Model file for the job. Use its own axes, mm. Coordinates: 2 decimals unless noted, no trailing zeros. Write each loop counter-clockwise with the first axis right and the second up, starting at its lowest first coordinate (ties: lowest second). Pieces come first, ordered by that corner, then holes.
Q1. Pin check, flat tip, straight feed: P1, Ø1, axis at x = 8, z = -2, coming from the +Y side. Stop position of the tip, or through.
Q2. Drill centre lines: probe 1 along X at (y, z) = (-1.3, 0); probe 2 along Z at (x, y) = (40, -1.3); probe 3 along X at (y, z) = (-1.5, -2). Where is each one in solid material? Low to high.
Q3. Band-saw the part on A-A, the plane x = -40. Write the cut outline in (y, z), plus the area to 3 significant figures.
Q4. Band-saw the part on B-B, the plane z = 0. Write the cut outline in (x, y).
Q5. Band-saw the part on C-C, the plane y = -1.1. Write the cut outline in (x, z), plus the area to 3 significant figures.
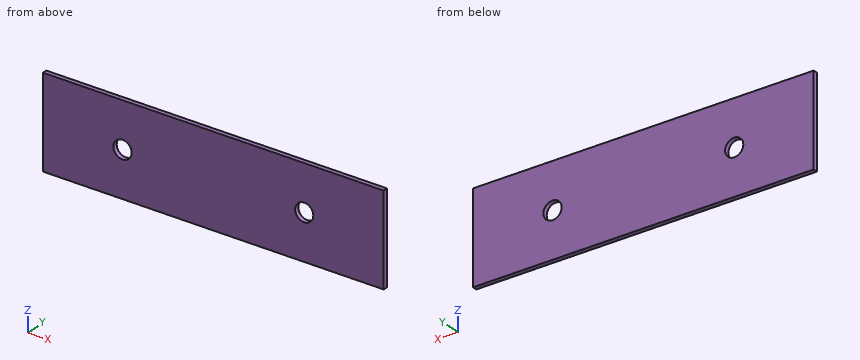
from build123d import *

# Parameters (mm, degrees)
SKETCH1_W          = 150
SKETCH1_H          = 40
BASE_FLANGE1_DEPTH = 2
SKETCH4_R          = 4
CUT_EXTRUDE1_DEPTH = 2


# Sheet-metal steps are written as plain solids
with BuildPart() as part:
    # Sketch1 → Base-Flange1 (new body)
    with BuildSketch(Plane(origin=(0, 0, 0), x_dir=(1, 0, 0), z_dir=(0, 1, 0))):
        Rectangle(SKETCH1_W, SKETCH1_H)
    extrude(amount=-BASE_FLANGE1_DEPTH)

    # Sketch4 → Cut-Extrude1 (cut)
    with BuildSketch(Plane(origin=(0, 0, 0), x_dir=(1, 0, 0), z_dir=(0, 1, 0))):
        with Locations(Location((-40, 0, 0), (0, 0, 270))):
            Circle(SKETCH4_R)
        with Locations(Location((40, 0, 0), (0, 0, 90))):
            Circle(SKETCH4_R)
    extrude(amount=-CUT_EXTRUDE1_DEPTH, mode=Mode.SUBTRACT)


solid = part.part
Answer sheet:
1. P1: stops at y = 0
2. probe 1: x = -75 to -44, -36 to 36, 44 to 75
2. probe 2: z = -20 to -4, 4 to 20
2. probe 3: x = -75 to -43.46, -36.54 to 36.54, 43.46 to 75
3. outline: (-2, -20) - (0, -20) - (0, -4) - (-2, -4) - close; (-2, 4) - (0, 4) - (0, 20) - (-2, 20) - close
3. area: 64.0 mm2
4. outline: (-75, -2) - (-44, -2) - (-44, 0) - (-75, 0) - close; (-36, -2) - (36, -2) - (36, 0) - (-36, 0) - close; (44, -2) - (75, -2) - (75, 0) - (44, 0) - close
5. outline: (-75, -20) - (75, -20) - (75, 20) - (-75, 20) - close; hole circle Ø8 at (-40, 0); hole circle Ø8 at (40, 0)
5. area: 5,900 mm2
